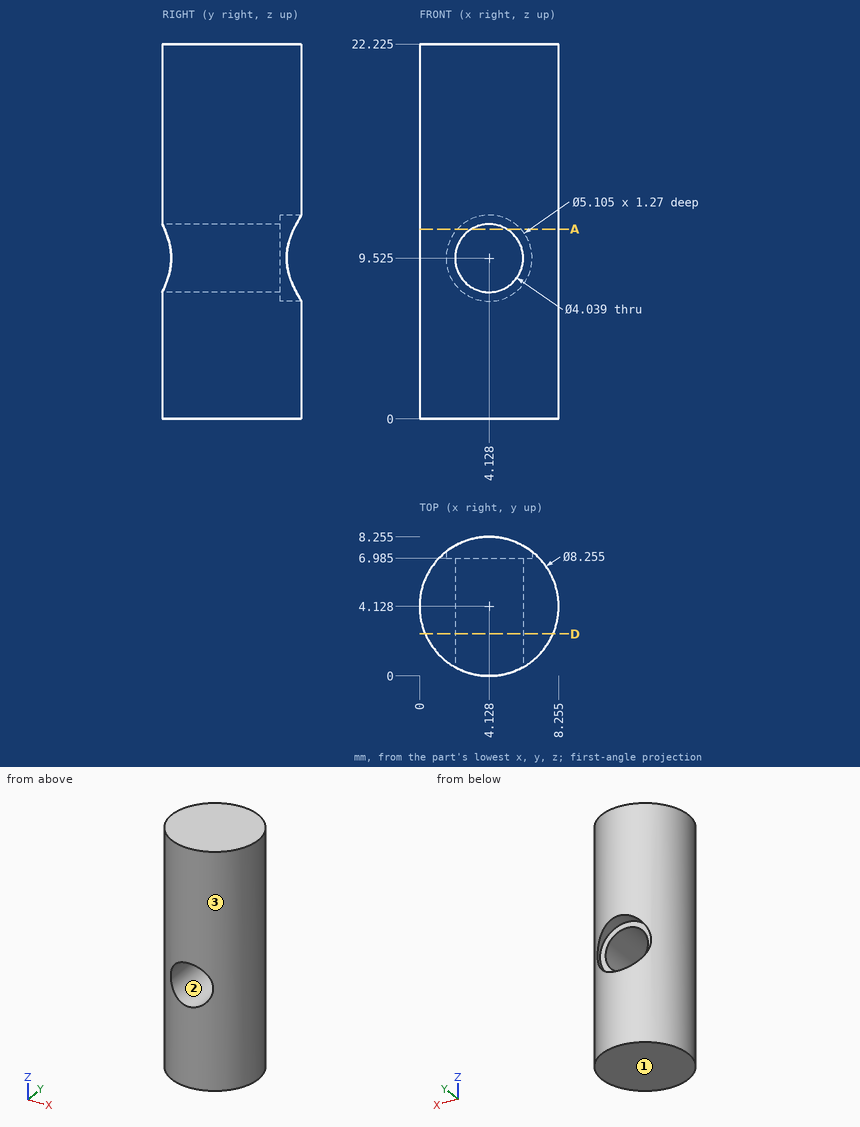
The figure shows three views and two pictorial views of one solid part (mm, origin at its lowest corner). Answer the questions. Give positions to 0.01 mm unless a question says otherwise; leave off trailing zeros. Loops run counter-clockwise (first coordinate to the right, second up) from the corner with the lowest first, then second, coordinate; pieces in that order, holes last. Notation, with made-up numbers: M 51,-21.5 L 66,-21.5 A17 ccw 66,-7.5 Z; hole C 79.25,70 d6. An arc over 180 degrees is marked long. Write each question's results on one line, items separated by ' | '.
1. The mould has two halves that part along X. Classify the marked faces 1, 2 and 3: pulls with the +X half, pulls with the -X half, needs draft (parallel to the pull), parting line crosses it, or undercut.
Values:
face 1: needs draft | face 2: undercut | face 3: parting line crosses it
2. Straight lines are drawn through the part: line 1 (Y direction, x = 4, z = 15.75); line 2 (X direction, y = 5.25, z = 9.5) (1 decimal). For each, find the intervals that lie inside material, in ascending order. Write a range as [from, to].
Values:
line 1: y = [0, 8.25] | line 2: x = [0.2, 2.1], [6.1, 8.1]
3. Section A-A on z = 11.25 is taken. Give the vertices of the cut face in (x, y) (1 decimal).
Values:
outline: M 2.2,7 L 2.2,7.8 A4.1 ccw 3.1,0.1 L 3.1,7 Z; M 5.2,0.1 A4.1 ccw 6,7.8 L 6,7 L 5.2,7 Z
4. Given pin 1 (4.5 mm diameter, centred on x = 4.13, z = 9.53, fed in from +Y) (1 decimal); pin 2 (1 mm diameter, centred on x = 7, z = 8.5, fed in from -Y), each flat-ended and moving along its own axis, determine where each tip first touches the part or whether it passes through.
Values:
pin 1: stops at y = 7 | pin 2: stops at y = 0.75
5. Section D-D on y = 2.5 is taken. Give the vertices of the cut face in (x, z) (1 decimal), plus the area to 3 significant figures.
Values:
outline: M 0.3,0 L 7.9,0 L 7.9,22.2 L 0.3,22.2 Z; hole C 4.1,9.5 d4 | area: 156 mm^2
